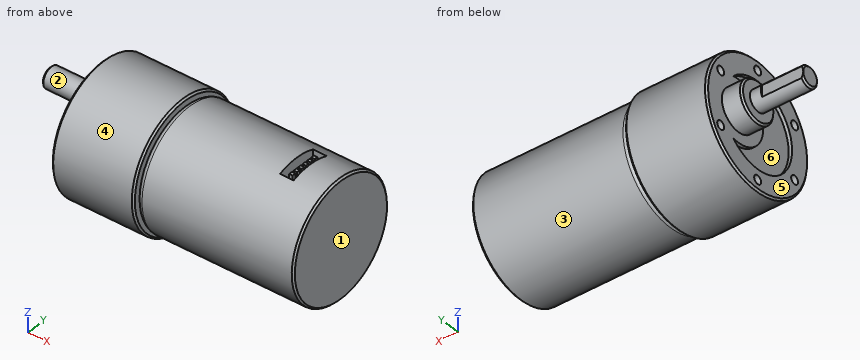
from build123d import *

# Parameters (mm, degrees)
SKETCH3_R                  = 6
BOSS_EXTRUDE1_DEPTH        = 5.8
SKETCH4_R                  = 3
BOSS_EXTRUDE2_DEPTH        = 15.2
SKETCH5_W                  = 3.31662479
SKETCH5_H                  = 2.173071946
CUT_EXTRUDE1_DEPTH         = 12
CHAMFER1_SIZE              = 0.5
CUT_EXTRUDE2_DEPTH         = 1
M3_TAPPED_HOLE1_AT_2_COUNT = 2
M3_TAPPED_HOLE1_AT_2_PITCH = 26.846787517
M3_TAPPED_HOLE1_AT_3_COUNT = 2
M3_TAPPED_HOLE1_AT_3_PITCH = 26.846787517
CIRPATTERN1_COUNT          = 2
SKETCH10_W                 = 4
SKETCH10_H                 = 12
CUT_EXTRUDE3_DEPTH         = 28
SKETCH11_W                 = 1
SKETCH11_H                 = 1
BOSS_EXTRUDE3_DEPTH        = 4
LPATTERN1_COUNT            = 6
LPATTERN1_PITCH            = 1.6


with BuildPart() as part:
    # Sketch1 → Revolve1 (revolve)
    with BuildSketch(Plane(origin=(0, 0, 0), x_dir=(1, 0, 0), z_dir=(0, 1, 0)), mode=Mode.PRIVATE) as revolve1_sk:
        with BuildLine():
            Line((0, 0), (69.8, 0))
            Line((69.8, 0), (69.8, 17.25))
            Line((69.8, 17.25), (25.5, 17.25))
            ThreePointArc((25.5, 17.25), (24.439339828, 16.810660172), (24, 15.75))
            Line((24, 15.75), (24, 18.5))
            Line((24, 18.5), (0, 18.5))
            Line((0, 18.5), (0, 0))
        make_face()
    revolve(revolve1_sk.sketch.rotate(Axis((0, 0, 0), (1, 0, 0)), 180), axis=Axis((0, 0, 0), (1, 0, 0)))

    # Sketch3 → Boss-Extrude1 (add)
    with BuildSketch(Plane.ZY):
        with Locations(Location((0, 7, 0), (0, 0, 180))):
            Circle(SKETCH3_R)
    extrude(amount=BOSS_EXTRUDE1_DEPTH)

    # Sketch4 → Boss-Extrude2 (add)
    with BuildSketch(Plane.ZY.offset(5.8)):
        with Locations(Location((0, 7, 0), (0, 0, 180))):
            Circle(SKETCH4_R)
    extrude(amount=BOSS_EXTRUDE2_DEPTH)

    # Sketch5 → Cut-Extrude1 (cut)
    with BuildSketch(Plane.ZY.offset(21)):
        with Locations((0, 10.586535973)):
            Rectangle(SKETCH5_W, SKETCH5_H)
    extrude(amount=-CUT_EXTRUDE1_DEPTH, mode=Mode.SUBTRACT)

    # Chamfer1
    chamfer1_edges = [part.edges().sort_by_distance(p)[0] for p in [
        (-5.8, 7, 6),
        (-21, 4.356617963, 1.418637165),
        (69.8, 0, -17.25),
        (24, 0, -18.5),
        (0, 0, -18.5),
    ]]
    chamfer(chamfer1_edges, length=CHAMFER1_SIZE - 0.0001)  # a hair under: the kernel refuses the full size

    # Sketch6 → Cut-Extrude2 (cut)
    with BuildSketch(Plane.ZY):
        with BuildLine():
            ThreePointArc((-8.802520946, 8.875), (0, -12.5), (8.802520946, 8.875))
            ThreePointArc((8.802520946, 8.875), (0, -2), (-8.802520946, 8.875))
        make_face()
    extrude(amount=-CUT_EXTRUDE2_DEPTH, mode=Mode.SUBTRACT)

    # Sketch8 → M3 Tapped Hole1 (revolve, cut)
    with BuildSketch(Plane(origin=(0, -13.423393759, -7.75), x_dir=(0, 0, 1), z_dir=(0, 1, 0))):
        Polygon((0, 0), (0, 4.751075774), (1.25, 4), (1.25, 0), align=None)
    m3_tapped_hole1 = revolve(axis=Axis((-6.35, -13.423393759, -7.75), (1, 0, 0)), mode=Mode.SUBTRACT)

    # M3 Tapped Hole1 at 2: M3 Tapped Hole1 ×2
    with Locations(*[(0, i * M3_TAPPED_HOLE1_AT_2_PITCH, 0) for i in range(1, M3_TAPPED_HOLE1_AT_2_COUNT)]):
        add(m3_tapped_hole1, mode=Mode.SUBTRACT)

    # M3 Tapped Hole1 at 3: M3 Tapped Hole1 ×2
    with Locations(*[Vector(0, 0.4999999999999991, 0.8660254037844392) * (i * M3_TAPPED_HOLE1_AT_3_PITCH) for i in range(1, M3_TAPPED_HOLE1_AT_3_COUNT)]):
        add(m3_tapped_hole1, mode=Mode.SUBTRACT)

    # CirPattern1: M3 Tapped Hole1 ×2 about axis
    cirpattern1_axis = Axis((0, 0, 0), (1, 0, 0))
    for i in range(1, CIRPATTERN1_COUNT):
        add(m3_tapped_hole1.rotate(cirpattern1_axis, i * 360 / CIRPATTERN1_COUNT), mode=Mode.SUBTRACT)

    # CirPattern1 copy 1 sketch → CirPattern1 copy 1 (revolve, cut)
    with BuildSketch(Plane(origin=(0, -13.423393759, 7.75), x_dir=(0, 0, -1), z_dir=(0, -1, 0))):
        Polygon((0, 0), (0, 4.751075774), (1.25, 4), (1.25, 0), align=None)
    revolve(axis=Axis((-6.35, -13.423393759, 7.75), (1, 0, 0)), mode=Mode.SUBTRACT)

    # CirPattern1 copy 2 sketch → CirPattern1 copy 2 (revolve, cut)
    with BuildSketch(Plane(origin=(0, 0, -15.5), x_dir=(0, 0, -1), z_dir=(0, -1, 0))):
        Polygon((0, 0), (0, 4.751075774), (1.25, 4), (1.25, 0), align=None)
    revolve(axis=Axis((-6.35, 0, -15.5), (1, 0, 0)), mode=Mode.SUBTRACT)

    # Sketch10 → Cut-Extrude3 (cut)
    with BuildSketch(Plane.XY.offset(40)):
        with Locations((58.8, 0)):
            Rectangle(SKETCH10_W, SKETCH10_H)
    extrude(amount=-CUT_EXTRUDE3_DEPTH, mode=Mode.SUBTRACT)

    # Sketch11 → Boss-Extrude3 (add)
    with BuildSketch(Plane.XY.offset(12)):
        with Locations((58.8, -4)):
            Rectangle(SKETCH11_W, SKETCH11_H)
    boss_extrude3 = extrude(amount=BOSS_EXTRUDE3_DEPTH)

    # LPattern1: Boss-Extrude3 ×6
    with Locations(*[(0, i * LPATTERN1_PITCH, 0) for i in range(1, LPATTERN1_COUNT)]):
        add(boss_extrude3)


solid = part.part
Design review of the part built by this model. Coordinates are the model's own, in mm. Face numbers are marked on the shaded views. A direction names the side the tool comes from. Coordinates: 2 decimals unless noted, no trailing zeros. Write each loop counter-clockwise with the first axis right and the second up, starting at its lowest first coordinate (ties: lowest second). Pieces come first, ordered by that corner, then holes. Notation, with made-up numbers: (69, 9.5) -> (121, 9.5) arc R37 ccw to (121, 48.5) -> close; hole circle Ø11 at (3.5, 7). An arc over 180 degrees is marked (long way). Write each question's results on one line, items separated by ' | '. Start each with the question number.
(1) Tool access review of the marked faces 1, 2 and 3: name each direction out of +Z, -Z, +X, -X, +Y, -Y from which nothing blocks a thin tool from reaching the whole face with its end or side.
(2) Clearance check with flat-ended pins moving along their axes: P1, Ø5, axis at y = 11.5, z = -6, coming from the -X side; P2, Ø2, axis at x = 56, z = -0.5, coming from the +Y side; P3, Ø4, axis at y = 0, z = -15.5, coming from the -X side; P4, Ø1, axis at x = -1.5, z = 8, coming from the +Y side. State where each tip first meets the part, or that it passes through.
(3) Take a section at B-B on x = -1. Write out the cut boundary in (y, z).
(4) Take a section at A-A on x = 34.5. Write out the cut boundary in (y, z).
(5) The part is to be moulded in two halves that separate along Z. For the marked faces 4, 5 and 6, say which applies: pulls with the +Z half, pulls with the -Z half, needs draft (parallel to the pull), parting line crosses it, or undercut.
(6) For line 1 along Y through (x, z) = (3, 7.75); line 2 along X through (y, z) = (-4, -2.5); line 3 along X through (y, z) = (8, 3), list the stretches that pass through material, from the lowest coordinate up. Write a range as from..to.
Results found:
1) face 1: +Z, -Z, +X, +Y, -Y | face 2: -X | face 3: +X
2) P1: stops at x = -5.8 | P2: stops at y = 17.25 | P3: stops at x = 0 | P4: passes through
3) outline: circle Ø12 at (7, 0)
4) outline: circle Ø34.5 at (0, 0)
5) face 4: parting line crosses it | face 5: needs draft | face 6: undercut
6) line 1: y = -16.8..-14.67, -12.17..12.17, 14.67..16.8 | line 2: x = 1..69.8 | line 3: x = -5.8..69.8
